from build123d import *

# Parameters (mm, degrees)
SKETCH1_W           = 6
SKETCH1_H           = 7
SKETCH1_H_2         = 29.5
SKETCH1_H_3         = 14
SKETCH1_H_4         = 13
BOSS_EXTRUDE1_DEPTH = 10
SKETCH1_4_W         = 6
SKETCH1_4_H         = 7
BOSS_EXTRUDE2_DEPTH = 10


with BuildPart() as part:
    # Sketch1 → Boss-Extrude1 (new body)
    with BuildSketch(Plane.XY):
        with BuildLine():
            Line((34.887222474, 175.012885516), (-15.022777526, 175.012885516))
            ThreePointArc((-15.022777526, 175.012885516), (-21.033185166, 172.523293156), (-23.522777526, 166.512885516))
            Line((-23.522777526, 166.512885516), (-23.522777526, 141.012885516))
            Line((-23.522777526, 141.012885516), (-17.522777526, 141.012885516))
            Line((-17.522777526, 141.012885516), (-17.522777526, 166.512885516))
            ThreePointArc((-17.522777526, 166.512885516), (-16.790544479, 168.280652469), (-15.022777526, 169.012885516))
            Line((-15.022777526, 169.012885516), (34.887222474, 169.012885516))
            ThreePointArc((34.887222474, 169.012885516), (36.657039007, 168.27860051), (37.387215745, 166.507085068))
            Line((37.387215745, 166.507085068), (37.347229203, 149.272885508))
            ThreePointArc((37.347229203, 149.272885508), (38.091175602, 147.476836668), (39.887222474, 146.732885516))
            Line((39.887222474, 146.732885516), (79.977222474, 146.732885516))
            ThreePointArc((79.977222474, 146.732885516), (81.744989427, 146.000652469), (82.477222474, 144.232885516))
            Line((82.477222474, 144.232885516), (82.477222474, 143.732885516))
            Line((82.477222474, 143.732885516), (88.477222474, 143.732885516))
            Line((88.477222474, 143.732885516), (88.477222474, 144.232885516))
            ThreePointArc((88.477222474, 144.232885516), (85.987630114, 150.243293156), (79.977222474, 152.732885516))
            Line((79.977222474, 152.732885516), (43.355273195, 152.732885516))
            Line((43.355273195, 152.732885516), (43.387199595, 166.493163991))
            ThreePointArc((43.387199595, 166.493163991), (40.904598686, 172.516316495), (34.887222474, 175.012885516))
        make_face()
        with Locations((-20.522777526, 137.512885516)):
            Rectangle(SKETCH1_W, SKETCH1_H)
        with Locations((-20.522777526, 119.262885516)):
            Rectangle(SKETCH1_W, SKETCH1_H_2)
        with Locations((-20.522777526, 101.012885516)):
            Rectangle(SKETCH1_W, SKETCH1_H)
        with BuildLine():
            ThreePointArc((-17.522777526, 71.512885516), (-16.790544479, 69.745118563), (-15.022777526, 69.012885516))
            Line((-15.022777526, 69.012885516), (79.977222474, 69.012885516))
            ThreePointArc((79.977222474, 69.012885516), (81.744989427, 69.745118563), (82.477222474, 71.512885516))
            Line((82.477222474, 71.512885516), (82.477222474, 95.732885516))
            Line((82.477222474, 95.732885516), (88.477222474, 95.732885516))
            Line((88.477222474, 95.732885516), (88.477222474, 71.512885516))
            ThreePointArc((88.477222474, 71.512885516), (85.987630114, 65.502477876), (79.977222474, 63.012885516))
            Line((79.977222474, 63.012885516), (-15.022777526, 63.012885516))
            ThreePointArc((-15.022777526, 63.012885516), (-21.033185166, 65.502477876), (-23.522777526, 71.512885516))
            Line((-23.522777526, 71.512885516), (-23.522777526, 97.512885516))
            Line((-23.522777526, 97.512885516), (-17.522777526, 97.512885516))
            Line((-17.522777526, 97.512885516), (-17.522777526, 71.512885516))
        make_face()
        with BuildLine():
            Line((82.477222474, 144.232885516), (82.477222474, 143.732885516))
            Line((82.477222474, 143.732885516), (82.477222474, 136.732885516))
            Line((82.477222474, 136.732885516), (82.477222474, 122.732885516))
            Line((82.477222474, 122.732885516), (82.477222474, 115.732885516))
            Line((82.477222474, 115.732885516), (82.477222474, 102.732885516))
            Line((82.477222474, 102.732885516), (82.477222474, 95.732885516))
            Line((82.477222474, 95.732885516), (82.477222474, 71.512885516))
            ThreePointArc((82.477222474, 71.512885516), (81.744989427, 69.745118563), (79.977222474, 69.012885516))
            Line((79.977222474, 69.012885516), (-15.022777526, 69.012885516))
            ThreePointArc((-15.022777526, 69.012885516), (-16.790544479, 69.745118563), (-17.522777526, 71.512885516))
            Line((-17.522777526, 71.512885516), (-17.522777526, 97.512885516))
            Line((-17.522777526, 97.512885516), (-17.522777526, 104.512885516))
            Line((-17.522777526, 104.512885516), (-17.522777526, 134.012885516))
            Line((-17.522777526, 134.012885516), (-17.522777526, 141.012885516))
            Line((-17.522777526, 141.012885516), (-17.522777526, 166.512885516))
            ThreePointArc((-17.522777526, 166.512885516), (-16.790544479, 168.280652469), (-15.022777526, 169.012885516))
            Line((-15.022777526, 169.012885516), (34.887222474, 169.012885516))
            ThreePointArc((34.887222474, 169.012885516), (36.657039007, 168.27860051), (37.387215745, 166.507085068))
            Line((37.387215745, 166.507085068), (37.347229203, 149.272885508))
            ThreePointArc((37.347229203, 149.272885508), (38.091175602, 147.476836668), (39.887222474, 146.732885516))
            Line((39.887222474, 146.732885516), (79.977222474, 146.732885516))
            ThreePointArc((79.977222474, 146.732885516), (81.744989427, 146.000652469), (82.477222474, 144.232885516))
        make_face()
        with Locations((85.477222474, 140.232885516)):
            Rectangle(SKETCH1_W, SKETCH1_H)
        with Locations((85.477222474, 129.732885516)):
            Rectangle(SKETCH1_W, SKETCH1_H_3)
        with Locations((85.477222474, 119.232885516)):
            Rectangle(SKETCH1_W, SKETCH1_H)
        with Locations((85.477222474, 109.232885516)):
            Rectangle(SKETCH1_W, SKETCH1_H_4)
        with Locations((85.477222474, 99.232885516)):
            Rectangle(SKETCH1_W, SKETCH1_H)
    extrude(amount=BOSS_EXTRUDE1_DEPTH)

    # Sketch1_4 → Boss-Extrude2 (add)
    with BuildSketch(Plane.XY):
        with Locations((85.477222474, 140.232885516)):
            Rectangle(SKETCH1_4_W, SKETCH1_4_H)
        with Locations((85.477222474, 119.232885516)):
            Rectangle(SKETCH1_4_W, SKETCH1_4_H)
        with Locations((85.477222474, 99.232885516)):
            Rectangle(SKETCH1_4_W, SKETCH1_4_H)
        with Locations((-20.522777526, 101.012885516)):
            Rectangle(SKETCH1_4_W, SKETCH1_4_H)
        with Locations((-20.522777526, 137.512885516)):
            Rectangle(SKETCH1_4_W, SKETCH1_4_H)
    extrude(amount=-BOSS_EXTRUDE2_DEPTH)


solid = part.part
Verification items for the finished model (mm, model axes). A direction names the side the tool comes from. Coordinates: 2 decimals unless noted, no trailing zeros. Order: outer loops, then holes, each group sorted by start corner. A loop starts at its lowest first (then second) coordinate and runs counter-clockwise, first axis right, second up. Notation, with made-up numbers: (16, 31) -> (20, 31) arc R15 ccw to (20, 45) -> close; hole circle Ø6 at (37, -38.5). An arc over 180 degrees is marked (long way). Put each result on its own line as item: value. Start each with the question number.
1. Cross-section at C-C, the plane x = 33. Record the boundary of the cut face in (y, z), then the cut area to 3 significant figures.
2. Access from +Z, -Z, +X, -X, +Y, -Y to the whole of each face (thin tool, end or side, straight path). Record for faces 5 (the flat face through (-17.523, 137, -5)), 6 (the flat face through (-21, 134.013, -5)), 7 (the flat face through (85, 102.733, -5)), 8 (the flat face through (85, 143.733, -5)).
3. Mould release check, pull along Y, two halves, no side actions. Record for faces 1 (the flat face through (85, 119, -10)), 2 (the flat face through (62, 152.733, 5)), 3 (the flat face through (85, 95.733, -5)), 4 (the flat face through (85, 122.733, -5)): released by +Y, released by -Y, zero draft, split by the parting line, or undercut.
4. Cross-section at B-B, the plane z = 6.5. Record the boundary of the cut face in (x, y), then the cut area to 3 significant figures.
5. Cross-section at D-D, the plane y = 89.5. Record the boundary of the cut face in (x, z), then the cut area to 3 significant figures.
6. Material ranges on L1, parallel to Z at x = 26.5, y = 146.5; L2, parallel to X at y = 99, z = -3.5; L3, parallel to Y at x = 61.5, z = 1.5, recorded low to high. Write a range as [from, to].
7. Go/stop test with flat-tipped pins: pin 1 Ø5 at (x, z) = (65.5, 5) entering from +Y; pin 2 Ø10 at (x, y) = (8, 128.5) entering from -Z; pin 3 Ø2 at (y, z) = (120.5, -7) entering from -X. Record where each tip stops, or that it passes through.
8. Cross-section at A-A, the plane z = -7.5. Record the boundary of the cut face in (x, y), then the cut area to 3 significant figures.
Computed:
1. outline: (63.01, 0) -> (175.01, 0) -> (175.01, 10) -> (63.01, 10) -> close
1. area: 1,120 mm2
2. face 5: -Z, +Y, -Y
2. face 6: -Z, +X, -X
2. face 7: -Z, +X
2. face 8: -Z, +X, -X, +Y
3. face 1: zero draft
3. face 2: released by +Y
3. face 3: released by -Y
3. face 4: undercut
4. outline: (-23.52, 71.51) arc R8.5 ccw to (-15.02, 63.01) -> (79.98, 63.01) arc R8.5 ccw to (88.48, 71.51) -> (88.48, 144.23) arc R8.5 ccw to (79.98, 152.73) -> (43.36, 152.73) -> (43.39, 166.49) arc R8.5 ccw to (34.89, 175.01) -> (-15.02, 175.01) arc R8.5 ccw to (-23.52, 166.51) -> close
4. area: 11,500 mm2
5. outline: (-23.52, 0) -> (88.48, 0) -> (88.48, 10) -> (-23.52, 10) -> close
5. area: 1,120 mm2
6. L1: [0, 10]
6. L2: [-23.52, -17.52], [82.48, 88.48]
6. L3: [63.01, 152.73]
7. pin 1: y = 152.73
7. pin 2: z = 0
7. pin 3: x = 82.48
8. outline: (-23.52, 97.51) -> (-17.52, 97.51) -> (-17.52, 104.51) -> (-23.52, 104.51) -> close; (-23.52, 134.01) -> (-17.52, 134.01) -> (-17.52, 141.01) -> (-23.52, 141.01) -> close; (82.48, 95.73) -> (88.48, 95.73) -> (88.48, 102.73) -> (82.48, 102.73) -> close; (82.48, 115.73) -> (88.48, 115.73) -> (88.48, 122.73) -> (82.48, 122.73) -> close; (82.48, 136.73) -> (88.48, 136.73) -> (88.48, 143.73) -> (82.48, 143.73) -> close
8. area: 210 mm2
